Work out the finished part from the listing and answer in its coordinate system (mm). A direction names the side the tool comes from. Give positions to 0.01 mm unless a question says otherwise; leave off trailing zeros. Order: outer loops, then holes, each group sorted by start corner. A loop starts at its lowest first (then second) coordinate and runs counter-clockwise, first axis right, second up. Notation, with made-up numbers: (3, -17) -> (53, -17) arc R38 cw to (53, 21) -> close; hole circle Ø10 at (13.5, -35). An arc over 180 degrees is marked (long way). Answer as CSV lines item,"result". Start each with the question number.
1. A cutting plane is placed at C-C (y = 27.5). Give the vertices of the cut face in (x, z).
2. For faces 5 (the cylindrical face through (14.366, 43.33, -0.521)), 6 (the flat face through (-24, 28.4, 0)), 7 (the flat face through (20, 33, 0)), determine the directions among +Z, -Z, +X, -X, +Y, -Y from which every point of the face is accessible in a straight line to the end or side of a thin tool.
3. A cutting plane is placed at A-A (x = 23.95). Give the vertices of the cut face in (y, z).
4. A cutting plane is placed at D-D (z = 9.25). Give the vertices of the cut face in (x, y).
5. For a pull along X with two mould halves and no side action, classify faces 1 (the cylindrical face through (21.998, 27.132, 4.566)), 2 (the flat face through (20, 13, 0)), 3 (the cylindrical face through (-22.598, 27.132, 3.526)), 4 (the flat face through (10, 48.4, 0)) as released by +X, released by -X, zero draft, split by the parting line, or undercut.
6. Flat-ended cylindrical pins translate along their axes: pin 1 (3 mm diameter, centred on y = 33.5, z = -1, fed in from -X); pin 2 (3.5 mm diameter, centred on x = 23, z = 0, fed in from +Y); pin 3 (5.5 mm diameter, centred on x = -22.5, z = -2, fed in from -Y); pin 4 (6.5 mm diameter, centred on x = 23.95, z = 5, fed in from -Y). Find the tip coordinate at first contact, or state that the pin passes through.
7. Find the intervals of material crossed by L1, parallel to X at y = 26.4, z = 5; L2, parallel to Y at x = -10, z = -4; L3, parallel to X at y = 12.5, z = -1, in increasing order.
8. A cutting plane is placed at B-B (z = 5). Give the vertices of the cut face in (x, y).
from build123d import *

# Parameters (mm, degrees)
SKETCH1_W           = 40
SKETCH1_H           = 20
BOSS_EXTRUDE1_DEPTH = 25.9
SKETCH2_W           = 54
SKETCH2_H           = 20
SKETCH2_R           = 2
BOSS_EXTRUDE2_DEPTH = 2.5
SKETCH3_W           = 40
SKETCH3_H           = 20
BOSS_EXTRUDE3_DEPTH = 10
SKETCH4_R           = 4
BOSS_EXTRUDE4_DEPTH = 10


with BuildPart() as part:
    # Sketch1 → Boss-Extrude1 (new body)
    with BuildSketch(Plane(origin=(0, 0, 0), x_dir=(1, 0, 0), z_dir=(0, 1, 0))):
        Rectangle(SKETCH1_W, SKETCH1_H)
    extrude(amount=BOSS_EXTRUDE1_DEPTH)

    # Sketch2 → Boss-Extrude2 (add)
    with BuildSketch(Plane(origin=(0, 25.9, 0), x_dir=(1, 0, 0), z_dir=(0, 1, 0))):
        Rectangle(SKETCH2_W, SKETCH2_H)
        with Locations(Location((-23.95, 5, 0), (0, 0, 270))):
            Circle(SKETCH2_R, mode=Mode.SUBTRACT)
        with Locations(Location((-23.95, -5, 0), (0, 0, 270))):
            Circle(SKETCH2_R, mode=Mode.SUBTRACT)
        with Locations(Location((23.95, 5, 0), (0, 0, 270))):
            Circle(SKETCH2_R, mode=Mode.SUBTRACT)
        with Locations(Location((23.95, -5, 0), (0, 0, 270))):
            Circle(SKETCH2_R, mode=Mode.SUBTRACT)
    extrude(amount=BOSS_EXTRUDE2_DEPTH)

    # Sketch3 → Boss-Extrude3 (add)
    with BuildSketch(Plane(origin=(0, 28.4, 0), x_dir=(1, 0, 0), z_dir=(0, 1, 0))):
        Rectangle(SKETCH3_W, SKETCH3_H)
    extrude(amount=BOSS_EXTRUDE3_DEPTH)

    # Sketch4 → Boss-Extrude4 (add)
    with BuildSketch(Plane(origin=(0, 38.4, 0), x_dir=(1, 0, 0), z_dir=(0, 1, 0))):
        with Locations(Location((10.4, 0, 0), (0, 0, 270))):
            Circle(SKETCH4_R)
    extrude(amount=BOSS_EXTRUDE4_DEPTH)


solid = part.part
Answer sheet:
1,outline,"(-27, -10) -> (27, -10) -> (27, 10) -> (-27, 10) -> close; hole circle Ø4 at (-23.95, -5); hole circle Ø4 at (-23.95, 5); hole circle Ø4 at (23.95, -5); hole circle Ø4 at (23.95, 5)"
2,face 5,"+Y"
2,face 6,"+Z, -Z, -X, +Y"
2,face 7,"+Z, -Z, +X, +Y"
3,outline,"(25.9, -10) -> (28.4, -10) -> (28.4, -7) -> (25.9, -7) -> close; (25.9, -3) -> (28.4, -3) -> (28.4, 3) -> (25.9, 3) -> close; (25.9, 7) -> (28.4, 7) -> (28.4, 10) -> (25.9, 10) -> close"
4,outline,"(-27, 25.9) -> (-20, 25.9) -> (-20, 0) -> (20, 0) -> (20, 25.9) -> (27, 25.9) -> (27, 28.4) -> (20, 28.4) -> (20, 38.4) -> (-20, 38.4) -> (-20, 28.4) -> (-27, 28.4) -> close"
5,face 1,"undercut"
5,face 2,"released by +X"
5,face 3,"undercut"
5,face 4,"zero draft"
6,pin 1,"stops at x = -20"
6,pin 2,"stops at y = 28.4"
6,pin 3,"stops at y = 0"
6,pin 4,"stops at y = 25.9"
7,L1,"x = -27 to -25.95, -21.95 to 21.95, 25.95 to 27"
7,L2,"y = 0 to 38.4"
7,L3,"x = -20 to 20"
8,outline,"(-27, 25.9) -> (-25.95, 25.9) -> (-25.95, 28.4) -> (-27, 28.4) -> close; (-21.95, 25.9) -> (-20, 25.9) -> (-20, 0) -> (20, 0) -> (20, 25.9) -> (21.95, 25.9) -> (21.95, 28.4) -> (20, 28.4) -> (20, 38.4) -> (-20, 38.4) -> (-20, 28.4) -> (-21.95, 28.4) -> close; (25.95, 25.9) -> (27, 25.9) -> (27, 28.4) -> (25.95, 28.4) -> close"
